```python
from build123d import *

# Parameters (mm, degrees)
SKETCH_1_R          = 4
EXTRUDE_1_DEPTH     = 2
SKETCH_2_R          = 10
EXTRUDE_2_DEPTH     = 2.5
SKETCH_3_R          = 1.6
CUT_EXTRUDE_1_DEPTH = 15.84082208


with BuildPart() as part:
    # 草图1 → 凸台-拉伸1 (new body)
    with BuildSketch(Plane(origin=(0, 0, 0), x_dir=(1, 0, 0), z_dir=(0, 1, 0))):
        with Locations(Location((0, 0, 0), (0, 0, 270))):
            Circle(SKETCH_1_R)
    extrude(amount=EXTRUDE_1_DEPTH)

    # 草图2 → 凸台-拉伸2 (add)
    with BuildSketch(Plane(origin=(0, 2, 0), x_dir=(1, 0, 0), z_dir=(0, 1, 0))):
        with Locations(Location((0, 0, 0), (0, 0, 270))):
            Circle(SKETCH_2_R)
    extrude(amount=EXTRUDE_2_DEPTH)

    # 草图3 → 切除-拉伸1 (cut, through all)
    with BuildSketch(Plane(origin=(0, 4.5, 0), x_dir=(1, 0, 0), z_dir=(0, 1, 0))):
        with Locations(Location((0, 0, 0), (0, 0, 270))):
            Circle(SKETCH_3_R)
        with Locations(Location((0, 7, 0), (0, 0, 270))):
            Circle(SKETCH_3_R)
        with Locations(Location((7, 0, 0), (0, 0, 270))):
            Circle(SKETCH_3_R)
        with Locations(Location((0, -7, 0), (0, 0, 270))):
            Circle(SKETCH_3_R)
        with Locations(Location((-7, 0, 0), (0, 0, 270))):
            Circle(SKETCH_3_R)
    extrude(amount=-CUT_EXTRUDE_1_DEPTH, mode=Mode.SUBTRACT)


solid = part.part
```
CAD build for the part. Positions are in the model's coordinates, mm. A direction names the side the tool comes from. Give positions to 0.01 mm unless a question says otherwise; leave off trailing zeros. Loops run counter-clockwise (first coordinate to the right, second up) from the corner with the lowest first, then second, coordinate; pieces in that order, holes last. Notation, with made-up numbers: M 76.25,48.25 L 83.25,48.25 A17 ccw 83.25,67.25 Z; hole C -34.75,26 d6. An arc over 180 degrees is marked long. Use one line per item in the form item = value.
Item 1: Two-plate mould, pull along X, no slides. Class faces 1 (the face through (-2, 4.5, 0)), 2 (the face through (-9.76, 3.23, -2.17)), 3 (the face through (5.44, 3.27, -0.35)): pulls with the +X half, pulls with the -X half, needs draft (parallel to the pull), parting line crosses it, or undercut.
Determined:
face_1 = needs draft
face_2 = parting line crosses it
face_3 = undercut
Item 2: Slice it at B-B (y = 2.3). List the corners of the cut face in (x, z).
Determined:
outline = C 0,0 d20; hole C -7,0 d3.2; hole C 0,-7 d3.2; hole C 0,0 d3.2; hole C 0,7 d3.2; hole C 7,0 d3.2
Item 3: Slice it at C-C (z = -7). List the corners of the cut face in (x, y), plus the area to 3 significant figures.
Determined:
outline = M -7.14,2 L -1.6,2 L -1.6,4.5 L -7.14,4.5 Z; M 1.6,2 L 7.14,2 L 7.14,4.5 L 1.6,4.5 Z
area = 27.7 mm2
Item 4: Slice it at A-A (x = 0). List the corners of the cut face in (y, z).
Determined:
outline = M 0,-4 L 2,-4 L 2,-5.4 L 4.5,-5.4 L 4.5,-1.6 L 0,-1.6 Z; M 0,1.6 L 4.5,1.6 L 4.5,5.4 L 2,5.4 L 2,4 L 0,4 Z; M 2,-10 L 4.5,-10 L 4.5,-8.6 L 2,-8.6 Z; M 2,8.6 L 4.5,8.6 L 4.5,10 L 2,10 Z
Item 5: Slice it at D-D (z = 0.5). List the corners of the cut face in (x, y).
Determined:
outline = M -9.99,2 L -8.52,2 L -8.52,4.5 L -9.99,4.5 Z; M -5.48,2 L -3.97,2 L -3.97,0 L -1.52,0 L -1.52,4.5 L -5.48,4.5 Z; M 1.52,0 L 3.97,0 L 3.97,2 L 5.48,2 L 5.48,4.5 L 1.52,4.5 Z; M 8.52,2 L 9.99,2 L 9.99,4.5 L 8.52,4.5 Z
Item 6: Which spindle directions (+Z, -Z, +X, -X, +Y, -Y) get a long thin tool onto all of the face, cutting with end or side? Do faces 4 (the face through (0.07, 3.27, 5.4)), 5 (the face through (0.1, 2, 4.3)). Say none if no direction does.
Determined:
face_4 = +Y, -Y
face_5 = -Y
Item 7: Drill centre lines: probe 1 along X at (y, z) = (1.2, 0); probe 2 along X at (y, z) = (2.05, 0); probe 3 along Y at (x, z) = (0.25, 9). Where is each one in solid material? Low to high. Write a range as from..to.
Determined:
probe_1 = -4..-1.6, 1.6..4
probe_2 = -10..-8.6, -5.4..-1.6, 1.6..5.4, 8.6..10
probe_3 = 2..4.5
Item 8: Flat gauge pins, fed straight in: pin 1 (2 mm diameter, centred on x = -2.5, z = 5.5, fed in from -Y); pin 2 (1.5 mm diameter, centred on y = 3, z = -4.5, fed in from +X). Where does each tip first touch, or does it go through?
Determined:
pin_1 = 2
pin_2 = 9.27
